```python
from build123d import *

# Parameters (mm, degrees)
ESBO_O1_R                = 4.5
RESSALTO_EXTRUS_O1_DEPTH = 3
ESBO_O2_R                = 3.25
RESSALTO_EXTRUS_O2_DEPTH = 12
ESBO_O3_R                = 2.5
RESSALTO_EXTRUS_O3_DEPTH = 4
FILETE2_R                = 0.3


with BuildPart() as part:
    # Esboço1 → Ressalto-extrusão1 (new body)
    with BuildSketch(Plane(origin=(0, 0, 0), x_dir=(1, 0, 0), z_dir=(0, 1, 0))):
        with Locations(Location((0, 0, 0), (0, 0, 270))):
            Circle(ESBO_O1_R)
    extrude(amount=RESSALTO_EXTRUS_O1_DEPTH)

    # Esboço2 → Ressalto-extrusão2 (add)
    with BuildSketch(Plane.XZ):
        with Locations(Location((0, 0, 0), (0, 0, 270))):
            Circle(ESBO_O2_R)
    extrude(amount=RESSALTO_EXTRUS_O2_DEPTH)

    # Esboço3 → Ressalto-extrusão3 (add)
    with BuildSketch(Plane.XZ.offset(12)):
        with Locations(Location((0, 0, 0), (0, 0, 270))):
            Circle(ESBO_O3_R)
    extrude(amount=RESSALTO_EXTRUS_O3_DEPTH)

    # Filete2
    filete2_edges = [part.edges().sort_by_distance(p)[0] for p in [
        (0, 0, -4.5),
    ]]
    fillet(filete2_edges, radius=FILETE2_R)


solid = part.part
```
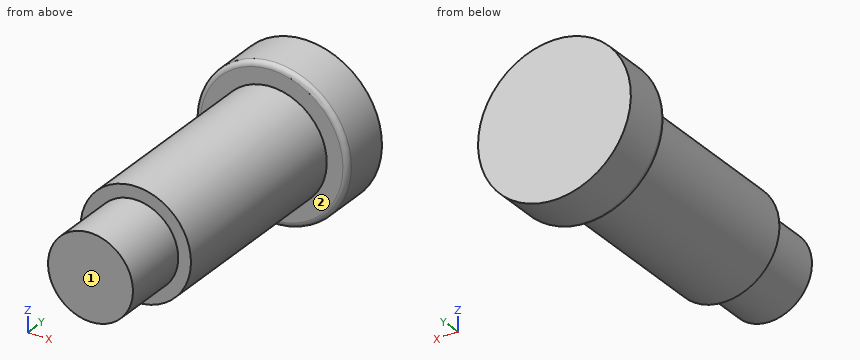
Here's how the part is built. I have some questions about the finished solid (model axes, mm). Face numbers are marked on the shaded views. A direction names the side the tool comes from. Round coordinates to 2 decimals unless told otherwise and drop trailing zeros. Write each loop counter-clockwise with the first axis right and the second up, starting at its lowest first coordinate (ties: lowest second). Pieces come first, ordered by that corner, then holes.
Q1. If we section it at D-D on y = -8.75: Write out the boundary of the cut face in (x, z), plus the area to 3 significant figures.
Q2. Please list where these lines run through material, in increasing order: probe 1 along Y at (x, z) = (-3.75, 0); probe 2 along Y at (x, z) = (3, -1); probe 3 along Z at (x, y) = (1, -14.75).
Q3. If we section it at B-B on x = 0: Write out the boundary of the cut face in (y, z).
Q4. If we section it at C-C on y = 1.75: Write out the boundary of the cut face in (x, z), plus the area to 3 significant figures.
Q5. Will these pins go through, and if not, where does the flat tip stop? P1, Ø4, axis at x = 2, y = -6.5, coming from the +Z side; P2, Ø1.5, axis at y = -12.5, z = 1, coming from the +X side; P3, Ø1.5, axis at y = -11, z = 3.5, coming from the +X side.
Q6. Which directions (+Z, -Z, +X, -X, +Y, -Y) give clear straight access to the entire face, cutting with the end or side of a thin tool? Please do the marked faces 1 and 2.
Q7. If we section it at A-A on z = 0: Write out the boundary of the cut face in (x, y), plus the area to 3 significant figures.
Answer below:
1. outline: circle Ø6.5 at (0, 0)
1. area: 33.2 mm2
2. probe 1: y = 0 to 3
2. probe 2: y = -12 to 3
2. probe 3: z = -2.29 to 2.29
3. outline: (-16, -2.5) - (-12, -2.5) - (-12, -3.25) - (0, -3.25) - (0, -4.2) arc R0.3 ccw to (0.3, -4.5) - (3, -4.5) - (3, 4.5) - (0.3, 4.5) arc R0.3 ccw to (0, 4.2) - (0, 3.25) - (-12, 3.25) - (-12, 2.5) - (-16, 2.5) - close
4. outline: circle Ø9 at (0, 0)
4. area: 63.6 mm2
5. P1: stops at z = 3.25
5. P2: stops at x = 3.22
5. P3: stops at x = 1.73
6. face 1: +Z, -Z, +X, -X, -Y
6. face 2: -Y
7. outline: (-4.5, 0.3) arc R0.3 ccw to (-4.2, 0) - (-3.25, 0) - (-3.25, -12) - (-2.5, -12) - (-2.5, -16) - (2.5, -16) - (2.5, -12) - (3.25, -12) - (3.25, 0) - (4.2, 0) arc R0.3 ccw to (4.5, 0.3) - (4.5, 3) - (-4.5, 3) - close
7. area: 125 mm2
